Design review of the part built by this model. Coordinates are the model's own, in mm. A direction names the side the tool comes from. Round coordinates to 2 decimals unless told otherwise and drop trailing zeros. Write each loop counter-clockwise with the first axis right and the second up, starting at its lowest first coordinate (ties: lowest second). Pieces come first, ordered by that corner, then holes.
from build123d import *

# Parameters (mm, degrees)
F0_R     = 3.75
F1_DEPTH = 8
F3_DEPTH = 2.5
F4_R     = 0.75
F5_DEPTH = 3
F7_DEPTH = 2


# Not quite as in the source:
# - a feature names something its author has since deleted; it is built from what else it names


with BuildPart() as f1:
    # F0 (on Front) → F1 (new body)
    with BuildSketch(Plane.XZ):
        Circle(F0_R)
    extrude(amount=F1_DEPTH)

    # F2 (on face) → F3 (join)
    with BuildSketch(Plane.XZ.offset(8)):
        with BuildLine():
            Line((-2.5, 1.6583123952), (-2.5, -1.6583123952))
            ThreePointArc((-2.5, -1.6583123952), (0, -3), (2.5, -1.6583123952))
            Line((2.5, -1.6583123952), (2.5, 1.6583123952))
            ThreePointArc((2.5, 1.6583123952), (0, 3), (-2.5, 1.6583123952))
        make_face()
    extrude(amount=F3_DEPTH)

    # F4 (on face) → F5 (join)
    with BuildSketch(Plane.XZ.offset(10.5)):
        Circle(F4_R)
    extrude(amount=F5_DEPTH)

    # F6 (on face) → F7 (join)
    with BuildSketch(Plane(origin=(0, 0, 0), x_dir=(-1, 0, 0), z_dir=(0, 1, 0))):
        with BuildLine():
            Line((0, 2.5), (-2.7950849719, 2.5))
            ThreePointArc((-2.7950849719, 2.5), (-3.75, 0), (-2.7950849719, -2.5))
            Line((-2.7950849719, -2.5), (0, -2.5))
            Line((0, -2.5), (0, 2.5))
        make_face()
        with BuildLine():
            Line((-2.7950849719, 2.5), (-5, 2.5))
            Line((-5, 2.5), (-5, -2.5))
            Line((-5, -2.5), (-2.7950849719, -2.5))
            ThreePointArc((-2.7950849719, -2.5), (-3.75, 0), (-2.7950849719, 2.5))
        make_face()
    extrude(amount=-F7_DEPTH)


solid = f1.part
1) Add section A-A on z = 0. State the section outline as (x, y) points, and give its area (3 significant figures).
2) Add section B-B on x = 0. State the section outline as (y, z) points, and give its area (3 significant figures).
3) Add section D-D on z = -2. State the section outline as (x, y) points, and give its area (3 significant figures).
4) For line 1 along Y through (x, z) = (1, -2.25); line 2 along Y through (x, z) = (2.5, -2.5); line 3 along X through (y, z) = (-4.5, 2.25), list the stretches that pass through material, from the lowest coordinate up.
5) For P1, Ø3, axis at y = -6.5, z = 0.5, coming from the +X side; P2, Ø0.6, axis at x = 4, y = -1.5, coming from the +Z side; P3, Ø1.5, axis at x = -2, y = -4, coming from the +Z side, all flat-tipped, find the tip position at first contact; note any pin that passes through.
6) Add section C-C on y = -11.5. State the section outline as (x, z) points.
7) For faces 1 (the face through (4, -1, -2.5)), 2 (the face through (0, -9, -3)), 3 (the face through (-3, -8, 0)), 4 (the face through (4, -1, 2.5)), 5 (the face through (0, -9, 3)), list the 3-axis set-ups (+Z, -Z, +X, -X, +Y, -Y) from which the entire face can be reached by the end or side of a thin tool; tool diameter is ignored.
Computed:
1. outline: (-3.75, -8) - (-2.5, -8) - (-2.5, -10.5) - (-0.75, -10.5) - (-0.75, -13.5) - (0.75, -13.5) - (0.75, -10.5) - (2.5, -10.5) - (2.5, -8) - (3.75, -8) - (3.75, -2) - (5, -2) - (5, 0) - (-3.75, 0) - close
1. area: 79.5 mm2
2. outline: (-13.5, -0.75) - (-10.5, -0.75) - (-10.5, -3) - (-8, -3) - (-8, -3.75) - (0, -3.75) - (0, 3.75) - (-8, 3.75) - (-8, 3) - (-10.5, 3) - (-10.5, 0.75) - (-13.5, 0.75) - close
2. area: 79.5 mm2
3. outline: (-3.17, -8) - (-2.24, -8) - (-2.24, -10.5) - (2.24, -10.5) - (2.24, -8) - (3.17, -8) - (3.17, -2) - (5, -2) - (5, 0) - (-3.17, 0) - close
3. area: 65.6 mm2
4. line 1: y = -10.5 to 0
4. line 2: y = -8 to 0
4. line 3: x = -3 to 3
5. P1: stops at x = 3.75
5. P2: stops at z = 2.5
5. P3: stops at z = 3.54
6. outline: circle Ø1.5 at (0, 0)
7. face 1: -Z, +X, +Y, -Y
7. face 2: -Z, -Y
7. face 3: -Y
7. face 4: +Z, +X, +Y, -Y
7. face 5: +Z, -Y
